Read the model definition and answer for the solid it produces. Units are mm, in the model's axes. A direction names the side the tool comes from. Round coordinates to 2 decimals unless told otherwise and drop trailing zeros. Order: outer loops, then holes, each group sorted by start corner. A loop starts at its lowest first (then second) coordinate and runs counter-clockwise, first axis right, second up. Notation, with made-up numbers: M -24,25 L 7,25 A6 cw 7,35 Z; hole C 51,-17.5 d8. An arc over 180 degrees is marked long. Answer as CSV lines item,"result".
Autodesk Inventor part; units mm, degrees
ref_plane "to_housing_XY" through (0, 0, 0) normal (0, 0, -1) x (1, 0, 0)
ref_plane "to_housing_YZ" through (0, 0, 0) normal (1, 0, 0) x (0, -1, 0)
ref_plane "to_housing_ZX" through (0, 0, 0) normal (0, -1, 0) x (0, 0, -1)
sketch "Sketch_1" plane through (0, 0, 0) normal (1, 0, 0) x (0, 0, -1)
  line L0 (5, 0) -> (0, 0)
  arc A0 (0, 4.7) -> (0.2, 4.5) centre (0.2, 4.7) ccw
  line L1 (0.2, 4.5) -> (4.8, 4.5)
  arc A1 (4.8, 4.5) -> (5, 4.7) centre (4.8, 4.7) ccw
  line L2 (5, 4.7) -> (5, 5.35)
  line L3 (5, 5.35) -> (4.8, 5.35)
  line L4 (4.8, 5.35) -> (4.8, 7.6)
  line L5 (4.8, 7.6) -> (5, 7.6)
  line L6 (5, 7.6) -> (5, 8.3)
  arc A2 (5, 8.3) -> (4.8, 8.5) centre (4.8, 8.3) ccw
  line L7 (4.8, 8.5) -> (0.2, 8.5)
  arc A3 (0.2, 8.5) -> (0, 8.3) centre (0.2, 8.3) ccw
  line L8 (0, 8.3) -> (0, 7.6)
  line L9 (0, 7.6) -> (0.2, 7.6)
  line L10 (0.2, 7.6) -> (0.2, 5.35)
  line L11 (0.2, 5.35) -> (0, 5.35)
  line L12 (0, 5.35) -> (0, 4.7)
revolve "Revolution1" add sketch "Sketch_1" angle 360 about axis through (0, 0, -5) along (0, 0, -1)
ref_plane "to_housing_XY" through (0, 0, 0) normal (0, 0, -1) x (1, 0, 0)
ref_plane "to_housing_YZ" through (0, 0, 0) normal (1, 0, 0) x (0, -1, 0)
ref_plane "to_housing_ZX" through (0, 0, 0) normal (0, -1, 0) x (0, 0, -1)
properties part number "SUTB689ZZ" material "ステンレス鋼"
Item 1: Determine the mould class of faces 1 (the face through (-5, 0, -5)), 2 (the face through (-7.167, 4.57, -2.468)), 3 (the face through (5.2, -1.8, -0.2)) for opening direction Y: +Y half, -Y half, draft (parallel to the pull), parting line (faces both ways), or undercut.
Ans:
face 1,"draft"
face 2,"parting line"
face 3,"undercut"
Item 2: Flat-ended cylindrical pins translate along their axes: pin 1 (1.5 mm diameter, centred on x = 5.5, z = -3.5, fed in from -Y); pin 2 (1.5 mm diameter, centred on y = -1.5, z = -4, fed in from -X). Find the tip coordinate at first contact, or state that the pin passes through.
Ans:
pin 1,"y = -7.05"
pin 2,"x = -8.47"
Item 3: A tool of negligible diameter and unlimited length cuts with its end or side. For faces 4 (the face through (-7, 4, -5)), 5 (the face through (5.2, -1.8, -4.8)), from which of +Z, -Z, +X, -X, +Y, -Y can it reach the whole face along a straight path? Write none if from no direction.
Ans:
face 4,"-Z, +X, -X, +Y, -Y"
face 5,"-Z"
Item 4: Find the intervals of material crossed by probe 1 along X at (y, z) = (0, -3.3); probe 2 along X at (y, z) = (0, -0.1); probe 3 along Z at (x, y) = (-7.5, 0.25), in increasing order. Write a range as [from, to].
Ans:
probe 1,"[-8.5, -4.5], [4.5, 8.5]"
probe 2,"[-8.47, -7.6], [-5.35, -4.53], [4.53, 5.35], [7.6, 8.47]"
probe 3,"[-4.8, -0.2]"
Item 5: A cutting plane is placed at C-C, the plane z = -3.55. Determine the outline of the cut face in (x, y).
Ans:
outline,"C 0,0 d17; hole C 0,0 d9"
